Read the model definition and answer for the solid it produces. Units are mm, in the model's axes. A direction names the side the tool comes from. Coordinates: 2 decimals unless noted, no trailing zeros. Order: outer loops, then holes, each group sorted by start corner. A loop starts at its lowest first (then second) coordinate and runs counter-clockwise, first axis right, second up. Notation, with made-up numbers: (28, -34) -> (51, -34) arc R31 ccw to (51, 0) -> close; hole circle Ø3 at (77, 74.25). An arc over 180 degrees is marked (long way). Return JSON: item names as keys, results as strings. Group by question number.
```python
from build123d import *

# Parameters (mm, degrees)
SKETCH1_R                                            = 16.5
BOSS_EXTRUDE1_DEPTH                                  = 4
CBORE_FOR_M3_HEX_SOCKET_THIN_HEAD_CAP_SC_D           = 3.4
CBORE_FOR_M3_HEX_SOCKET_THIN_HEAD_CAP_SC_CBORE_D     = 6.5
CBORE_FOR_M3_HEX_SOCKET_THIN_HEAD_CAP_SC_CBORE_DEPTH = 2.4
F_3_0MM_DOWEL_HOLE1_D                                = 3
F_3_0MM_DOWEL_HOLE1_DEPTH                            = 6
F_3_0MM_DOWEL_HOLE1_TIP                              = 0.901290929
TAP_DRILL_FOR_M3_HELICOIL1_D                         = 3.15


with BuildPart() as part:
    # Sketch1 → Boss-Extrude1 (new body)
    with BuildSketch(Plane(origin=(0, 0, 0), x_dir=(1, 0, 0), z_dir=(0, 1, 0))):
        with Locations(Location((0, 0, 0), (0, 0, 270))):
            Circle(SKETCH1_R)
    extrude(amount=BOSS_EXTRUDE1_DEPTH)

    # CBORE for M3 Hex Socket Thin Head Cap Screw1 (through all)
    with Locations(Plane.XZ):
        with Locations((0, 0)):
            CounterBoreHole(CBORE_FOR_M3_HEX_SOCKET_THIN_HEAD_CAP_SC_D / 2, CBORE_FOR_M3_HEX_SOCKET_THIN_HEAD_CAP_SC_CBORE_D / 2, CBORE_FOR_M3_HEX_SOCKET_THIN_HEAD_CAP_SC_CBORE_DEPTH)

    # Ø3.0mm Dowel Hole1
    with Locations(Plane(origin=(0, 0, 0), x_dir=(-1, 0, 0), z_dir=(0, -1, 0))):
        with Locations((-10.825317547, -6.25), (0, 12.5), (10.825317547, -6.25)):
            Hole(F_3_0MM_DOWEL_HOLE1_D / 2, depth=F_3_0MM_DOWEL_HOLE1_DEPTH)
            with Locations((0, 0, -(F_3_0MM_DOWEL_HOLE1_DEPTH + F_3_0MM_DOWEL_HOLE1_TIP / 2))):  # 118° drill point
                Cone(0, F_3_0MM_DOWEL_HOLE1_D / 2, F_3_0MM_DOWEL_HOLE1_TIP, mode=Mode.SUBTRACT)

    # Tap Drill for M3 Helicoil1 (through all)
    with Locations(Plane(origin=(0, 0, 0), x_dir=(-1, 0, 0), z_dir=(0, -1, 0))):
        with Locations((10.825317547, 6.25), (0, -12.5), (-10.825317547, 6.25)):
            Hole(TAP_DRILL_FOR_M3_HELICOIL1_D / 2)


solid = part.part
```
1. Find section B-B on y = 1.9. Determine the outline of the cut face in (x, z) (3 decimals), and give its area (3 significant figures).
2. Straight lines are drawn through the part: L1, parallel to X at y = 1.7, z = 5.5; L2, parallel to X at y = 2.05, z = 6.25; L3, parallel to Y at x = -2, z = 2. For each, find the intervals that lie inside material, in ascending order.
3. Which of the six approach directions +Z, -Z, +X, -X, +Y, -Y give full straight-line access (tool end or side, diameter ignored) to faces 4 (the face through (-9.44, 2.03, 6.82)), 5 (the face through (1.4, 2.4, -1.4))?
4. Given pin 1 (1 mm diameter, centred on y = 3, z = -5, fed in from +X); pin 2 (2 mm diameter, centred on y = 0.5, z = -9.5, fed in from +X); pin 3 (2 mm diameter, centred on x = 11, y = 0.5, fed in from -Z), each flat-ended and moving along its own axis, determine where each tip first touches the part or whether it passes through.
5. Find section C-C on z = 5.5. Determine the outline of the cut face in (x, y).
6. Find section D-D on y = 3.55. Determine the outline of the cut face in (x, z) (3 decimals).
7. Find section A-A on z = 0. Determine the outline of the cut face in (x, y), and give its area (3 significant figures).
8. For a pull along Z with two mould halves and no side action, classify faces 1 (the face through (-16.108, 1.972, -3.577)), 2 (the face through (0.2, 0, 3.4)), 3 (the face through (-9.98, 2.03, -7.58)) as released by +Z, released by -Z, zero draft, split by the parting line, or undercut.
Result:
{
 "1": {"outline": "circle Ø33 at (0, 0); hole circle Ø3.15 at (-10.825, -6.25); hole circle Ø3 at (-10.825, 6.25); hole circle Ø6.5 at (0, 0); hole circle Ø3.15 at (0, 12.5); hole circle Ø3 at (0, -12.5); hole circle Ø3.15 at (10.825, -6.25); hole circle Ø3 at (10.825, 6.25)", "area": "778 mm^2"},
 "2": {"L1": "-15.56 to -12.12, -9.53 to 9.53, 12.12 to 15.56", "L2": "-15.27 to -12.33, -9.33 to 9.33, 12.33 to 15.27", "L3": "2.4 to 4"},
 "3": {"face 4": "+Y, -Y", "face 5": "-Y"},
 "4": {"pin 1": "x = 15.87", "pin 2": "x = 14.14", "pin 3": "z = -13.12"},
 "5": {"outline": "(-15.56, 0) -> (-12.12, 0) -> (-12.12, 4) -> (-15.56, 4) -> close; (-9.53, 0) -> (9.53, 0) -> (9.53, 4) -> (-9.53, 4) -> close; (12.12, 0) -> (15.56, 0) -> (15.56, 4) -> (12.12, 4) -> close"},
 "6": {"outline": "circle Ø33 at (0, 0); hole circle Ø3.15 at (-10.825, -6.25); hole circle Ø3 at (-10.825, 6.25); hole circle Ø3.4 at (0, 0); hole circle Ø3.15 at (0, 12.5); hole circle Ø3 at (0, -12.5); hole circle Ø3.15 at (10.825, -6.25); hole circle Ø3 at (10.825, 6.25)"},
 "7": {"outline": "(-16.5, 0) -> (-3.25, 0) -> (-3.25, 2.4) -> (-1.7, 2.4) -> (-1.7, 4) -> (-16.5, 4) -> close; (1.7, 2.4) -> (3.25, 2.4) -> (3.25, 0) -> (16.5, 0) -> (16.5, 4) -> (1.7, 4) -> close", "area": "111 mm^2"},
 "8": {"face 1": "split by the parting line", "face 2": "zero draft", "face 3": "undercut"}
}
